The listing builds one solid part. Answer for the finished solid, in the listing's coordinates (mm). Face numbers are marked on the shaded views. A direction names the side the tool comes from. Coordinates: 2 decimals unless noted, no trailing zeros. Write each loop counter-clockwise with the first axis right and the second up, starting at its lowest first coordinate (ties: lowest second). Pieces come first, ordered by that corner, then holes. Notation, with made-up numbers: M -23.5,55 L 8.5,55 A23 cw 8.5,80 Z; hole C -38.75,-12 d11. An arc over 180 degrees is marked long. Answer as a JSON object with one key per item and string values. Group by question number.
from build123d import *

# Parameters (mm, degrees)
ESQUISSE1_W                                       = 100
ESQUISSE1_H                                       = 80
BOSS_EXTRU_1_DEPTH                                = 10
ESQUISSE2_W                                       = 70
ESQUISSE2_H                                       = 80
BOSS_EXTRU_2_DEPTH                                = 12
BOSS_EXTRU_3_DEPTH                                = 6.15
ESQUISSE3_W                                       = 8
ESQUISSE3_H                                       = 4
CHAMBRAGE_POUR_VIS_SIX_PANS_CREUX_M41_D           = 4.5
CHAMBRAGE_POUR_VIS_SIX_PANS_CREUX_M41_CBORE_D     = 8
CHAMBRAGE_POUR_VIS_SIX_PANS_CREUX_M41_CBORE_DEPTH = 4.4
ENL_V_MAT_EXTRU_1_DEPTH                           = 134.812639538
CONG_1_R                                          = 2


with BuildPart() as part:
    # Esquisse1 → Boss.-Extru.1 (new body)
    with BuildSketch(Plane(origin=(0, 0, 0), x_dir=(1, 0, 0), z_dir=(0, 1, 0))):
        with Locations((-50, 40)):
            Rectangle(ESQUISSE1_W, ESQUISSE1_H)
    extrude(amount=BOSS_EXTRU_1_DEPTH)

    # Esquisse2 → Boss.-Extru.2 (add)
    with BuildSketch(Plane(origin=(0, 10, 0), x_dir=(1, 0, 0), z_dir=(0, 1, 0))):
        with Locations((-50, 40)):
            Rectangle(ESQUISSE2_W, ESQUISSE2_H)
    extrude(amount=BOSS_EXTRU_2_DEPTH)

    # Esquisse7 → Boss.-Extru.3 (add)
    with BuildSketch(Plane(origin=(0, 0, -80), x_dir=(-1, 0, 0), z_dir=(0, 0, -1))):
        with BuildLine():
            Line((70, 22), (30, 22))
            ThreePointArc((30, 22), (50, 2), (70, 22))
        make_face()
    extrude(amount=BOSS_EXTRU_3_DEPTH)

    # Esquisse3 → Enlèvement de matière-Révolution1 (revolve, cut)
    with BuildSketch(Plane(origin=(0, 22, 0), x_dir=(1, 0, 0), z_dir=(0, 1, 0))):
        Polygon((-37.8, 82.15), (-50, 82.15), (-50, 75.95), (-42, 75.95), (-37.8, 75.95), align=None)
        with Locations((-46, 73.95)):
            Rectangle(ESQUISSE3_W, ESQUISSE3_H)
        Polygon((-42, 71.95), (-50, 71.95), (-50, 14.2), (-42, 14.2), (-28.5, 14.2), (-28.5, 71.95), align=None)
        with Locations((-46, 12.2)):
            Rectangle(ESQUISSE3_W, ESQUISSE3_H)
        Polygon((-42, 10.2), (-50, 10.2), (-50, 4), (-42, 4), (-37.8, 4), (-37.8, 10.2), align=None)
        with Locations((-46, 2)):
            Rectangle(ESQUISSE3_W, ESQUISSE3_H)
    revolve(axis=Axis((-50, 22, -86.15), (0, 0, 1)), mode=Mode.SUBTRACT)

    # Chambrage pour vis à six pans creux M41 (through all)
    with Locations(Plane(origin=(-92.5, 10, -70), x_dir=(0, 0, 1), z_dir=(0, 1, 0))):
        with Locations((0, 0), (60, 0), (60, 85), (0, 85)):
            CounterBoreHole(CHAMBRAGE_POUR_VIS_SIX_PANS_CREUX_M41_D / 2, CHAMBRAGE_POUR_VIS_SIX_PANS_CREUX_M41_CBORE_D / 2, CHAMBRAGE_POUR_VIS_SIX_PANS_CREUX_M41_CBORE_DEPTH)

    # Esquisse6 → Enlèv. mat.-Extru.1 (cut, through all)
    with BuildSketch(Plane.XY):
        with BuildLine():
            Line((-15, 22), (-18, 22))
            Line((-18, 22), (-18, 13.656854249))
            ThreePointArc((-18, 13.656854249), (-18.617316568, 12.732974717), (-19.707106781, 12.949747468))
            Line((-19.707106781, 12.949747468), (-22.535533906, 15.778174593))
            ThreePointArc((-22.535533906, 15.778174593), (-23.242640687, 16.071067812), (-23.949747468, 15.778174593))
            Line((-23.949747468, 15.778174593), (-24.656854249, 15.071067812))
            ThreePointArc((-24.656854249, 15.071067812), (-24.949747468, 14.363961031), (-24.656854249, 13.656854249))
            Line((-24.656854249, 13.656854249), (-18.292893219, 7.292893219))
            ThreePointArc((-18.292893219, 7.292893219), (-17.96846987, 7.076120467), (-17.585786438, 7))
            Line((-17.585786438, 7), (-16, 7))
            ThreePointArc((-16, 7), (-15.292893219, 7.292893219), (-15, 8))
            Line((-15, 8), (-15, 9))
            ThreePointArc((-15, 9), (-14.707106781, 9.707106781), (-14, 10))
            Line((-14, 10), (-15, 10))
            Line((-15, 10), (-15, 22))
        make_face()
        with BuildLine():
            Line((-82, 13.656854249), (-82, 22))
            Line((-82, 22), (-85, 22))
            Line((-85, 22), (-85, 10))
            Line((-85, 10), (-86, 10))
            ThreePointArc((-86, 10), (-85.292893219, 9.707106781), (-85, 9))
            Line((-85, 9), (-85, 8))
            ThreePointArc((-85, 8), (-84.707106781, 7.292893219), (-84, 7))
            Line((-84, 7), (-82.414213562, 7))
            ThreePointArc((-82.414213562, 7), (-82.03153013, 7.076120467), (-81.707106781, 7.292893219))
            Line((-81.707106781, 7.292893219), (-75.343145751, 13.656854249))
            ThreePointArc((-75.343145751, 13.656854249), (-75.050252532, 14.363961031), (-75.343145751, 15.071067812))
            Line((-75.343145751, 15.071067812), (-76.050252532, 15.778174593))
            ThreePointArc((-76.050252532, 15.778174593), (-76.757359313, 16.071067812), (-77.464466094, 15.778174593))
            Line((-77.464466094, 15.778174593), (-80.292893219, 12.949747468))
            ThreePointArc((-80.292893219, 12.949747468), (-81.382683432, 12.732974717), (-82, 13.656854249))
        make_face()
    extrude(amount=-ENL_V_MAT_EXTRU_1_DEPTH, mode=Mode.SUBTRACT)

    # Congé1
    # the kernel refuses this fillet: 2 mm, written as the material it adds along each edge
    with BuildSketch(Plane(origin=(-50, 22, -80), x_dir=(1, 0, 0), z_dir=(0, 1, 0))) as cong_1_piece_1:
        with BuildLine():
            CenterArc((20 + CONG_1_R, CONG_1_R), CONG_1_R, 180, 90)
            Line((20, CONG_1_R), (20, 0))
            Line((20, 0), (20 + CONG_1_R, 0))
        make_face()
    revolve(axis=Axis((-50, 22, -80), (0, 0, -1)), revolution_arc=180)
    # the kernel refuses this fillet: 2 mm, written as the material it takes off along each edge
    with BuildSketch(Plane(origin=(-2, 8, -78), x_dir=(0, 1, 0), z_dir=(0, 0, -1))) as cong_1_2_piece_1_section:
        Polygon((0, 0), (CONG_1_R * 1.02, 0), (CONG_1_R * 1.02, CONG_1_R * 1.02), (0, CONG_1_R * 1.02), align=None)
    cong_1_2_piece_1 = extrude(amount=CONG_1_R * 1.02, mode=Mode.PRIVATE)
    cong_1_2_piece_1 = cong_1_2_piece_1 - Plane(origin=(-2, 8, -78), x_dir=(-0.7071067811865475, -0.7071067811865475, 0), z_dir=(0, 0, -1)) * Sphere(CONG_1_R, mode=Mode.PRIVATE)
    add(cong_1_2_piece_1, mode=Mode.SUBTRACT)
    with BuildSketch(Plane(origin=(-98, 8, -78), x_dir=(-1, 0, 0), z_dir=(0, 0, -1))) as cong_1_2_piece_2_section:
        Polygon((0, 0), (CONG_1_R * 1.02, 0), (CONG_1_R * 1.02, CONG_1_R * 1.02), (0, CONG_1_R * 1.02), align=None)
    cong_1_2_piece_2 = extrude(amount=CONG_1_R * 1.02, mode=Mode.PRIVATE)
    cong_1_2_piece_2 = cong_1_2_piece_2 - Plane(origin=(-98, 8, -78), x_dir=(0.7071067811865475, -0.7071067811865475, 0), z_dir=(0, 0, -1)) * Sphere(CONG_1_R, mode=Mode.PRIVATE)
    add(cong_1_2_piece_2, mode=Mode.SUBTRACT)
    with BuildSketch(Plane(origin=(-2, 8, -2), x_dir=(0, 1, 0), z_dir=(0, 0, 1))) as cong_1_2_piece_3_section:
        Polygon((0, 0), (CONG_1_R * 1.02, 0), (CONG_1_R * 1.02, -CONG_1_R * 1.02), (0, -CONG_1_R * 1.02), align=None)
    cong_1_2_piece_3 = extrude(amount=CONG_1_R * 1.02, mode=Mode.PRIVATE)
    cong_1_2_piece_3 = cong_1_2_piece_3 - Plane(origin=(-2, 8, -2), x_dir=(-0.7071067811865475, -0.7071067811865475, 0), z_dir=(0, 0, 1)) * Sphere(CONG_1_R, mode=Mode.PRIVATE)
    add(cong_1_2_piece_3, mode=Mode.SUBTRACT)
    with BuildSketch(Plane(origin=(-98, 8, -2), x_dir=(-1, 0, 0), z_dir=(0, 0, 1))) as cong_1_2_piece_4_section:
        Polygon((0, 0), (CONG_1_R * 1.02, 0), (CONG_1_R * 1.02, -CONG_1_R * 1.02), (0, -CONG_1_R * 1.02), align=None)
    cong_1_2_piece_4 = extrude(amount=CONG_1_R * 1.02, mode=Mode.PRIVATE)
    cong_1_2_piece_4 = cong_1_2_piece_4 - Plane(origin=(-98, 8, -2), x_dir=(0.7071067811865475, -0.7071067811865475, 0), z_dir=(0, 0, 1)) * Sphere(CONG_1_R, mode=Mode.PRIVATE)
    add(cong_1_2_piece_4, mode=Mode.SUBTRACT)
    with BuildSketch(Plane(origin=(0, -5, -80), x_dir=(0, 0, 1), z_dir=(0, 1, 0)), Plane(origin=(0, -5, 0), x_dir=(-1, 0, 0), z_dir=(0, 1, 0))) as cong_1_2_piece_5:
        with BuildLine():
            CenterArc((CONG_1_R, -CONG_1_R), CONG_1_R, 90, 90)
            Line((0, -CONG_1_R), (0, 0))
            Line((0, 0), (CONG_1_R, 0))
        make_face()
    extrude(amount=13, mode=Mode.SUBTRACT)
    with BuildSketch(Plane(origin=(-100, -5, -80), x_dir=(0, 0, 1), z_dir=(0, 1, 0)), Plane(origin=(-100, -5, 0), x_dir=(1, 0, 0), z_dir=(0, 1, 0))) as cong_1_2_piece_6:
        with BuildLine():
            CenterArc((CONG_1_R, CONG_1_R), CONG_1_R, 180, 90)
            Line((0, CONG_1_R), (0, 0))
            Line((0, 0), (CONG_1_R, 0))
        make_face()
    extrude(amount=13, mode=Mode.SUBTRACT)
    with BuildSketch(Plane(origin=(0, 10, -78), x_dir=(-1, 0, 0), z_dir=(0, 0, 1))) as cong_1_2_piece_7:
        with BuildLine():
            CenterArc((CONG_1_R, CONG_1_R), CONG_1_R, 180, 90)
            Line((0, CONG_1_R), (0, 0))
            Line((0, 0), (CONG_1_R, 0))
        make_face()
    extrude(amount=76, mode=Mode.SUBTRACT)
    with BuildSketch(Plane(origin=(-2, 10, 0), x_dir=(0, -1, 0), z_dir=(-1, 0, 0)), Plane(origin=(-81, 10, 0), x_dir=(0, -1, 0), z_dir=(-1, 0, 0))) as cong_1_2_piece_8:
        with BuildLine():
            CenterArc((CONG_1_R, -CONG_1_R), CONG_1_R, 90, 90)
            Line((0, -CONG_1_R), (0, 0))
            Line((0, 0), (CONG_1_R, 0))
        make_face()
    extrude(amount=17, mode=Mode.SUBTRACT)
    with BuildSketch(Plane(origin=(-100, 10, -2), x_dir=(0, -1, 0), z_dir=(0, 0, -1))) as cong_1_2_piece_9:
        with BuildLine():
            CenterArc((CONG_1_R, -CONG_1_R), CONG_1_R, 90, 90)
            Line((0, -CONG_1_R), (0, 0))
            Line((0, 0), (CONG_1_R, 0))
        make_face()
    extrude(amount=76, mode=Mode.SUBTRACT)
    with BuildSketch(Plane(origin=(-19, 10, -80), x_dir=(0, 0, 1), z_dir=(1, 0, 0)), Plane(origin=(-98, 10, -80), x_dir=(0, 0, 1), z_dir=(1, 0, 0))) as cong_1_2_piece_10:
        with BuildLine():
            CenterArc((CONG_1_R, CONG_1_R), CONG_1_R, 180, 90)
            Line((0, CONG_1_R), (0, 0))
            Line((0, 0), (CONG_1_R, 0))
        make_face()
    extrude(amount=17, mode=Mode.SUBTRACT)
    with BuildSketch(Plane(origin=(-50, 22, -86.15), x_dir=(0.9688128753181994, 0.24779348784357297, 0), z_dir=(-0.24779348784357297, 0.9688128753181994, 0))) as cong_1_2_piece_11:
        with BuildLine():
            CenterArc((20 - CONG_1_R, -CONG_1_R), CONG_1_R, 0, 90)
            Line((20 - CONG_1_R, 0), (20, 0))
            Line((20, 0), (20, -CONG_1_R))
        make_face()
    revolve(axis=Axis((-50, 22, -86.15), (0, 0, -1)), revolution_arc=208.69396098, mode=Mode.SUBTRACT)


solid = part.part
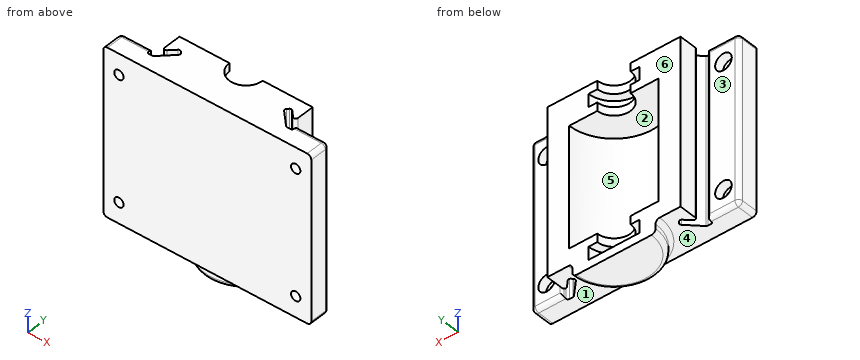
Item 1: A cutting plane is placed at B-B, the plane z = -70. State how many separate pieces and enclosed holes the cut face has, and give its area (3 significant figures).
Item 2: A tool of negligible diameter and unlimited length cuts with its end or side. For the marked faces 1, 2 and 3, from which of +Z, -Z, +X, -X, +Y, -Y can it reach the whole face along a straight path? Write none if from no direction.
Item 3: For a pull along Z with two mould halves and no side action, classify the marked faces 4, 5 and 6 as +Z half, -Z half, draft (parallel to the pull), parting line (faces both ways), or undercut.
Item 4: Consider L1, parallel to X at y = 7.5, z = -10; L2, parallel to Z at x = -58, y = 8.75; L3, parallel to Y at x = -6.5, z = -37.5. Determine where each line is inside the solid, lowest interval first. Write a range as from..to.
Item 5: Flat-ended cylindrical pins translate along their axes: pin 1 Ø10.5 at (x, z) = (-92.5, -70) entering from +Y; pin 2 Ø4 at (y, z) = (17.5, -57.5) entering from -X; pin 3 Ø2.5 at (x, z) = (-6.5, -10.5) entering from +Y. Find the tip coordinate at first contact, or state that the pin passes through.
Item 6: A cutting plane is placed at A-A, the plane x = -7.5. Write down the section's boundary in (y, z), and give its area (3 significant figures).
Answer:
{
 "1": {"separate pieces": "3", "enclosed holes": "0", "area": "846 mm2"},
 "2": {"face 1": "-Z, +X, -Y", "face 2": "+Y", "face 3": "+Z, -Z, -X, +Y"},
 "3": {"face 4": "-Z half", "face 5": "undercut", "face 6": "draft"},
 "4": {"L1": "-100..-96.5, -88.5..-84.87, -81.5..-18.5, -15.13..-11.5, -3.5..0", "L2": "-86.15..-71.95, -14.2..0", "L3": "0..10"},
 "5": {"pin 1": "y = 10", "pin 2": "x = -82", "pin 3": "y = 5.6"},
 "6": {"outline": "M 0,-80 L 8,-80 A2 ccw 10,-78 L 10,-74 L 5.6,-74 L 5.6,-72.25 L 0,-72.25 Z; M 0,-67.75 L 5.6,-67.75 L 5.6,-66 L 10,-66 L 10,-14 L 5.6,-14 L 5.6,-12.25 L 0,-12.25 Z; M 0,-7.75 L 5.6,-7.75 L 5.6,-6 L 10,-6 L 10,-2 A2 ccw 8,0 L 0,0 Z", "area": "677 mm2"}
}
